from build123d import *

# Parameters (mm, degrees)
M8_GEWINDEBOHRUNG1_D            = 6.8
M8_GEWINDEBOHRUNG1_DEPTH        = 22.25
M8_GEWINDEBOHRUNG1_CSINK_D      = 9
M8_GEWINDEBOHRUNG1_CSINK_ANGLE  = 60
M8_GEWINDEBOHRUNG1_TIP          = 2.042926105
FASE1_SIZE                      = 1
FASE1_SIZE2                     = 0.577350269
SCHNITT_LINEAR_AUSTRAGEN1_DEPTH = 4


with BuildPart() as part:
    # Skizze1 → Rotation1 (revolve)
    with BuildSketch(Plane(origin=(0, 0, 0), x_dir=(1, 0, 0), z_dir=(0, 1, 0))):
        Polygon((0, 0), (0, 12.5), (95, 12.5), (95, 12.4), (125, 12.4), (125, 12.5), (149.133974596, 12.5), (150, 12), (150, 0), align=None)
    revolve(axis=Axis((0, 0, 0), (-1, 0, 0)))

    # Skizze3 → Schnitt-Rotation1 (revolve, cut)
    with BuildSketch(Plane(origin=(150, 0, 0), x_dir=(0, 0, -1), z_dir=(0, -1, 0)), mode=Mode.PRIVATE) as schnitt_rotation1_sk:
        Polygon((0, -5.351075774), (1.25, -4.6), (1.25, -2.424871131), (2.65, 0), (0, 0), align=None)
    revolve(schnitt_rotation1_sk.sketch.rotate(Axis((150, 0, 0), (-1, 0, 0)), 270), axis=Axis((150, 0, 0), (-1, 0, 0)), mode=Mode.SUBTRACT)

    # M8 Gewindebohrung1
    with Locations(Plane.ZY):
        with Locations((0, 0)):
            CounterSinkHole(M8_GEWINDEBOHRUNG1_D / 2, M8_GEWINDEBOHRUNG1_CSINK_D / 2, depth=M8_GEWINDEBOHRUNG1_DEPTH, counter_sink_angle=M8_GEWINDEBOHRUNG1_CSINK_ANGLE)
            with Locations((0, 0, -(M8_GEWINDEBOHRUNG1_DEPTH + M8_GEWINDEBOHRUNG1_TIP / 2))):  # 118° drill point
                Cone(0, M8_GEWINDEBOHRUNG1_D / 2, M8_GEWINDEBOHRUNG1_TIP, mode=Mode.SUBTRACT)

    # Fase1
    fase1_edges = [part.edges().sort_by_distance(p)[0] for p in [
        (0, 0, 12.5),
    ]]
    fase1_side = [part.faces().sort_by_distance(p)[0] for p in [
        (47.5, 0, 12.5),
    ]]
    chamfer(fase1_edges, length=FASE1_SIZE, length2=FASE1_SIZE2, reference=fase1_side[0])

    # Skizze2 → Schnitt-Linear austragen1 (cut)
    with BuildSketch(Plane(origin=(0, 12.5, 4.921019115), x_dir=(1, 0, 0), z_dir=(0, 1, 0))):
        with BuildLine():
            Line((14, 8.921019115), (56, 8.921019115))
            ThreePointArc((56, 8.921019115), (60, 4.921019115), (56, 0.921019115))
            Line((56, 0.921019115), (14, 0.921019115))
            ThreePointArc((14, 0.921019115), (10, 4.921019115), (14, 8.921019115))
        make_face()
    extrude(amount=-SCHNITT_LINEAR_AUSTRAGEN1_DEPTH, mode=Mode.SUBTRACT)


solid = part.part
Here's how the part is built. I have some questions about the finished solid (model axes, mm). A direction names the side the tool comes from. Coordinates: 2 decimals unless noted, no trailing zeros. Order: outer loops, then holes, each group sorted by start corner. A loop starts at its lowest first (then second) coordinate and runs counter-clockwise, first axis right, second up. Notation, with made-up numbers: M 42.25,21 L 90.25,21 A30 cw 90.25,45 Z; hole C -15.75,0.25 d3. An arc over 180 degrees is marked long. Answer as CSV lines item,"result". Start each with the question number.
1. On a 3-axis mill with a long thin cutter (end or side, diameter ignored), from which of +Z, -Z, +X, -X, +Y, -Y can I reach the whole of each face in a straight line? I mean faces 1 (the cylindrical face through (110.21, 11, -5.72)), 2 (the cylindrical face through (137.236, -3.755, -11.923)), 3 (the cylindrical face through (60, 11, 0)). Say none if no direction works.
2. I want a section at B-B, the plane x = 133. Write out the boundary of the cut face in (y, z).
3. I need wall thicknesses on line 1 (Y direction, x = 12, z = 0); line 2 (Z direction, x = 15.25, y = 0); line 3 (Z direction, x = 146.85, y = 0). Which ranges of each line are inside material? Lowest first, please. Write a range as [from, to].
4. I want a section at A-A, the plane x = 44.5. Write out the boundary of the cut face in (y, z).
5. We'd pull the mould along Y, two halves only. Please class faces 4 (the flat face through (35, 10, 4)), 5 (the cylindrical face through (12.22, -3.32, 0.74)), 6 (the cylindrical face through (146.5, -0.27, 1.22)), 7 (the flat face through (35, 8.5, 0)): released by +Y, released by -Y, zero draft, split by the parting line, or undercut.
6. For pin 1 (3 mm diameter, centred on y = 0, z = 0, fed in from -X); pin 2 (9 mm diameter, centred on x = 45.5, z = -2, fed in from +Y); pin 3 (10 mm diameter, centred on x = 101.5, y = -10, fed in from +Z), each with a flat end and sliding along its axis, tell me the tip position at first contact or that it passes through.
Recorded:
1,face 1,"none"
1,face 2,"+X, -X"
1,face 3,"+Y"
2,outline,"C 0,0 d25"
3,line 1,"y = [-12.5, -3.4], [3.4, 8.5]"
3,line 2,"z = [-12.5, -3.4], [3.4, 12.5]"
3,line 3,"z = [-12.5, -1.25], [1.25, 12.5]"
4,outline,"M 8.5,-4 L 8.5,4 L 11.84,4 A12.5 ccw long 11.84,-4 Z"
5,face 4,"zero draft"
5,face 5,"undercut"
5,face 6,"undercut"
5,face 7,"released by +Y"
6,pin 1,"stops at x = 23.39"
6,pin 2,"stops at y = 11.84"
6,pin 3,"stops at z = 11.35"
